Input: part model. Units: mm. Frame: model coordinates. Face numbers are marked on the shaded views. A direction names the side the tool comes from. Coordinates: 2 decimals unless noted, no trailing zeros. Loops run counter-clockwise (first coordinate to the right, second up) from the corner with the lowest first, then second, coordinate; pieces in that order, holes last. Notation, with made-up numbers: (-34.5, -0.75) - (-26.5, -0.75) arc R20 ccw to (-26.5, 30.25) - close; hole circle Ø9 at (84.25, 57.25). An arc over 180 degrees is marked (long way). Use a Markdown table: item, result. Add a question column.
1. Section query B-B on y = 81. Return the cut outline in (x, z).
2. Access query for the marked faces 1, 2, 3 and 4. Directions: +Z, -Z, +X, -X, +Y, -Y. A direction counts if a zero-diameter tool reaches every point of the face in a straight line with its end or side. Return the directions, or none.
3. Section query D-D on x = -3. Return the cut outline in (y, z), then the cut area to 3 significant figures.
4. Section query C-C on z = -13. Return the cut outline in (x, y), then the cut area to 3 significant figures.
5. Contact query for flat-ended pins moving along their axis: P1, Ø17, axis at y = 61, z = -38.5, coming from the +X side; P2, Ø19.5, axis at x = 55.5, y = 58.5, coming from the +Z side; P3, Ø5, axis at x = 17, y = 39.5, coming from the +Z side; P4, Ø5, axis at x = -18, y = 31, coming from the +Z side. Output: stop coordinate, or through.
6. Section query A-A on z = -25. Return the cut outline in (x, y).
7. Ray query, L1, parallel to Y at x = 54, z = -33; L2, parallel to X at y = -0.5, z = -30.5; L3, parallel to Y at x = -17, z = -27.5. Return the intervals inside material, ascending. Write a range as [from, to].
8. Draft query along Y for the marked faces 5, 6 and 7. Return one class per face: released by +Y, released by -Y, zero draft, split by the parting line, or undercut.
```python
from build123d import *

# Parameters (mm, degrees)
Y_KSEKLIK_EKSTR_ZYON1_DEPTH = 52
IZIM3_R                     = 9
Y_KSEKLIK_EKSTR_ZYON2_DEPTH = 34
FEDER1_REACH                = 139.277
IZIM4_WALL_W                = 408.307741914
IZIM4_WALL_H                = 22


with BuildPart() as part:
    # Çizim1 → Yükseklik-Ekstrüzyon1 (new body)
    with BuildSketch(Plane.XY):
        with BuildLine():
            Line((-54, 34), (54, 34))
            ThreePointArc((54, 34), (88, 0), (54, -34))
            Line((54, -34), (-54, -34))
            ThreePointArc((-54, -34), (-88, 0), (-54, 34))
        make_face()
        with BuildLine():
            Line((-54, 15), (54, 15))
            ThreePointArc((54, 15), (69, 0), (54, -15))
            Line((54, -15), (-54, -15))
            ThreePointArc((-54, -15), (-69, 0), (-54, 15))
        make_face(mode=Mode.SUBTRACT)
    extrude(amount=-Y_KSEKLIK_EKSTR_ZYON1_DEPTH)

    # Çizim3 → Yükseklik-Ekstrüzyon2 (add)
    with BuildSketch(Plane.XY.offset(-18)):
        with BuildLine():
            ThreePointArc((79, 76), (54, 101), (29, 76))
            Line((29, 76), (29, 49))
            ThreePointArc((29, 49), (24.606601718, 38.393398282), (14, 34))
            Line((14, 34), (54, 34))
            ThreePointArc((54, 34), (67.647767834, 31.140623519), (79, 23.043437244))
            Line((79, 23.043437244), (79, 76))
        make_face()
        with Locations((54, 76)):
            Circle(IZIM3_R, mode=Mode.SUBTRACT)
    extrude(amount=-Y_KSEKLIK_EKSTR_ZYON2_DEPTH)

    # Çizim4 wall → Feder1 (add, up to next)
    with BuildSketch(Plane(origin=(-15.293433294, 63.226194681, -30), x_dir=(0.855125243419, 0.518421467599, 0), z_dir=(-0.518421467599, 0.855125243419, 0)), mode=Mode.PRIVATE) as feder1_sk1:
        with Locations((0, 11)):
            Rectangle(IZIM4_WALL_W, IZIM4_WALL_H)
    feder1_tool1 = extrude(feder1_sk1.sketch, amount=-FEDER1_REACH, mode=Mode.PRIVATE) - part.part
    add(feder1_tool1.solids().sort_by_distance((-15.293433294, 63.226194681, -30))[0])


solid = part.part
```
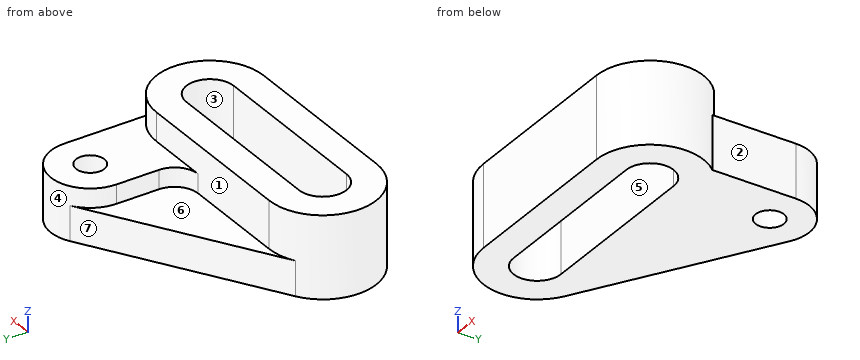
Resolved:
| question | item | result |
|---|---|---|
| 1 | outline | (14.02, -52) - (46.52, -52) - (46.52, -18) - (29.51, -18) - (29.51, -30) - (14.02, -30) - close; (61.48, -52) - (78.49, -52) - (78.49, -18) - (61.48, -18) - close |
| 2 | face 1 | +Z, -X, +Y |
| 2 | face 2 | +Z, -Z, +X, +Y |
| 2 | face 3 | +Z, -Z |
| 2 | face 4 | +Z, +Y |
| 3 | outline | (-34, -52) - (-15, -52) - (-15, 0) - (-34, 0) - close; (15, -52) - (70.68, -52) - (70.68, -30) - (34, -30) - (34, 0) - (15, 0) - close |
| 3 | area | 2,780 mm² |
| 4 | outline | (-54, -34) - (54, -34) arc R34 ccw to (54, 34) - (-54, 34) arc R34 ccw to start; hole (-54, -15) - (54, -15) arc R15 ccw to (54, 15) - (-54, 15) arc R15 ccw to start |
| 4 | area | 7,030 mm² |
| 5 | P1 | x = 79 |
| 5 | P2 | z = -18 |
| 5 | P3 | z = -30 |
| 5 | P4 | z = 0 |
| 6 | outline | (-54, -34) - (54, -34) arc R34 ccw to (79, 23.04) - (79, 76) arc R25 ccw to (29, 76) - (29, 49) arc R15 cw to (14, 34) - (-54, 34) arc R34 ccw to start; hole (-54, -15) - (54, -15) arc R15 ccw to (54, 15) - (-54, 15) arc R15 ccw to start; hole circle Ø18 at (54, 76) |
| 7 | L1 | [-34, -15], [15, 67], [85, 101] |
| 7 | L2 | [-88, -68.99], [68.99, 88] |
| 7 | L3 | [-34, -15], [15, 34] |
| 8 | face 5 | undercut |
| 8 | face 6 | zero draft |
| 8 | face 7 | released by +Y |
